from build123d import *

# Parameters (mm, degrees)
ESBO_O1_W                = 51.2
ESBO_O1_H                = 51.2
ESBO_O1_W_2              = 50
ESBO_O1_H_2              = 50
RESSALTO_EXTRUS_O1_DEPTH = 50
ESBO_O2_W                = 51.2
ESBO_O2_H                = 51.2
RESSALTO_EXTRUS_O2_DEPTH = 0.6
ESBO_O3_R                = 5.5
CORTE_EXTRUS_O1_DEPTH    = 0.6
ESBO_O4_R                = 2.5
CORTE_EXTRUS_O2_DEPTH    = 77.401308889
CORTE_EXTRUS_O3_REACH    = 78.401
ESBO_O5_R                = 2.5


with BuildPart() as part:
    # Esboço1 → Ressalto-extrusão1 (new body)
    with BuildSketch(Plane.XY):
        Rectangle(ESBO_O1_W, ESBO_O1_H)
        Rectangle(ESBO_O1_W_2, ESBO_O1_H_2, mode=Mode.SUBTRACT)
    extrude(amount=RESSALTO_EXTRUS_O1_DEPTH)

    # Esboço2 → Ressalto-extrusão2 (add)
    with BuildSketch(Plane.XY.offset(50)):
        Rectangle(ESBO_O2_W, ESBO_O2_H)
    extrude(amount=RESSALTO_EXTRUS_O2_DEPTH)

    # Esboço3 → Corte-extrusão1 (cut)
    with BuildSketch(Plane(origin=(25.6, 0, 0), x_dir=(0, 0, -1), z_dir=(1, 0, 0))):
        with Locations((-30.6, -7.6)):
            Circle(ESBO_O3_R)
    extrude(amount=-CORTE_EXTRUS_O1_DEPTH, mode=Mode.SUBTRACT)

    # Esboço4 → Corte-extrusão2 (cut, through all)
    with BuildSketch(Plane(origin=(25.6, 0, 0), x_dir=(0, 0, -1), z_dir=(1, 0, 0))):
        with Locations((-15, 0)):
            Circle(ESBO_O4_R)
    extrude(amount=-CORTE_EXTRUS_O2_DEPTH, mode=Mode.SUBTRACT)

    # Esboço5 → Corte-extrusão3 (cut, up to next)
    with BuildSketch(Plane.XZ.offset(25.6), mode=Mode.PRIVATE) as corte_extrus_o3_sk1:
        with Locations(Location((0, 38.6, 0), (0, 0, 270))):
            Circle(ESBO_O5_R)
    corte_extrus_o3_tool1 = extrude(corte_extrus_o3_sk1.sketch, amount=-CORTE_EXTRUS_O3_REACH, mode=Mode.PRIVATE) & part.part
    add(corte_extrus_o3_tool1.solids().sort_by_distance((0, -25.6, 38.6))[0], mode=Mode.SUBTRACT)


solid = part.part
Geometry check sheet. Reference: the model listing, model coordinates, mm. A direction names the side the tool comes from. Give positions to 0.01 mm unless a question says otherwise; leave off trailing zeros. Loops run counter-clockwise (first coordinate to the right, second up) from the corner with the lowest first, then second, coordinate; pieces in that order, holes last.
(1) Section check A-A on y = 0. Record the cut outline in (x, z).
From the geometry:
outline: (-25.6, 0) - (-25, 0) - (-25, 12.5) - (-25.6, 12.5) - close; (-25.6, 17.5) - (-25, 17.5) - (-25, 50) - (25, 50) - (25, 17.5) - (25.6, 17.5) - (25.6, 50.6) - (-25.6, 50.6) - close; (25, 0) - (25.6, 0) - (25.6, 12.5) - (25, 12.5) - close
(2) Thickness scan on L1, parallel to X at y = 7.5, z = 13.5; L2, parallel to Y at x = -25.2, z = 15. Record the ranges inside material, lowest first.
From the geometry:
L1: x = -25.6 to -25, 25 to 25.6
L2: y = -25.6 to -2.5, 2.5 to 25.6
(3) Section check B-B on x = 0. Record the cut outline in (y, z).
From the geometry:
outline: (-25.6, 0) - (-25, 0) - (-25, 36.1) - (-25.6, 36.1) - close; (-25.6, 41.1) - (-25, 41.1) - (-25, 50) - (25, 50) - (25, 0) - (25.6, 0) - (25.6, 50.6) - (-25.6, 50.6) - close
(4) Set-up check for faces 4 (the flat face through (-25, 0, 25)), 5 (the cylindrical face through (25.304, -7.358, 36.095)), 6 (the cylindrical face through (-0.96, -25.3, 36.29)), 7 (the flat face through (0, -25.6, 25)): record each of +Z, -Z, +X, -X, +Y, -Y from which the full face is reachable in a straight line by a thin tool's end or side.
From the geometry:
face 4: -Z
face 5: +X
face 6: -Y
face 7: +Z, -Z, +X, -X, -Y
(5) Section check D-D on z = 4. Record the cut outline in (x, y).
From the geometry:
outline: (-25.6, -25.6) - (25.6, -25.6) - (25.6, 25.6) - (-25.6, 25.6) - close; hole (-25, -25) - (25, -25) - (25, 25) - (-25, 25) - close
(6) Section check C-C on y = -7.6. Record the cut outline in (x, z), then the cut area to 3 significant figures.
From the geometry:
outline: (-25.6, 0) - (-25, 0) - (-25, 50) - (25, 50) - (25, 36.1) - (25.6, 36.1) - (25.6, 50.6) - (-25.6, 50.6) - close; (25, 0) - (25.6, 0) - (25.6, 25.1) - (25, 25.1) - close
area: 84.1 mm2
(7) Release check for a two-part mould opening along Z. For faces 1 (the flat face through (0, 25, 25)), 2 (the flat face through (0, 0, 50)), 3 (the cylindrical face through (-25.3, 0.1, 17.5)) record: released by +Z, released by -Z, zero draft, split by the parting line, or undercut.
From the geometry:
face 1: zero draft
face 2: released by -Z
face 3: undercut
(8) Depth check by flat-ended pin: pin 1 Ø5 at (x, y) = (-2, -4.5) entering from -Z; pin 2 Ø3 at (x, z) = (0, 38.6) entering from -Y. Enter the tip coordinate at first touch or a pass-through.
From the geometry:
pin 1: stops at z = 50
pin 2: stops at y = 25
